Verification items for the finished model (mm, model axes). A direction names the side the tool comes from. Give positions to 0.01 mm unless a question says otherwise; leave off trailing zeros. Order: outer loops, then holes, each group sorted by start corner. A loop starts at its lowest first (then second) coordinate and runs counter-clockwise, first axis right, second up.
(1) Gauge pin test, flat end, axial feed: pin 1 (1.4 mm diameter, centred on x = -2.67, z = -1.24, fed in from -Y). Record the tip position at first contact, or that the pin passes through.
(2) Access from +Z, -Z, +X, -X, +Y, -Y to the whole of each face (thin tool, end or side, straight path). Record for faces 4 (the face through (-8, 2, -3.388)), 5 (the face through (-12.598, 2, 4)).
(3) Sectioned sample at B-B on z = 3. Record the cut outline in (x, y), plus the area to 3 significant figures.
(4) Sectioned sample at A-A on x = -9.5. Record the cut outline in (y, z), plus the area to 3 significant figures.
(5) Mould release check, pull along Z, two halves, no side actions. Record for faces 1 (the face through (-6, 5, 4)), 2 (the face through (-6, 2, -4.541)), 3 (the face through (-8.17, 2.46, 1.41)): pulls with the +Z half, pulls with the -Z half, needs draft (parallel to the pull), parting line crosses it, or undercut.
(6) Sectioned sample at C-C on y = 4.2. Record the cut outline in (x, z).
(7) Scan lines: L1, parallel to Z at x = -4, y = 3.6; L2, parallel to X at y = 2.8, z = 3.5; L3, parallel to X at y = 2.95, z = 9. Record each from-to range of solid material in increasing order.
```python
from build123d import *

# Parameters (mm, degrees)
SKETCH1_W           = 13.581948161
SKETCH1_H           = 17.761009134
SKETCH1_R           = 1.6
SKETCH1_R_2         = 1.2
SKETCH1_R_3         = 1.75
BOSS_EXTRUDE1_DEPTH = 5


with BuildPart() as part:
    # Sketch1 → Boss-Extrude1 (new body)
    with BuildSketch(Plane(origin=(0, 0, 0), x_dir=(1, 0, 0), z_dir=(0, 1, 0))):
        with Locations((-5.80679888, -4.339957405)):
            Rectangle(SKETCH1_W, SKETCH1_H)
        with Locations(Location((-2.596056365, -9.056132184, 0), (0, 0, 270))):
            Circle(SKETCH1_R, mode=Mode.SUBTRACT)
        with Locations(Location((-2.667047062, 1.237786047, 0), (0, 0, 270))):
            Circle(SKETCH1_R_2, mode=Mode.SUBTRACT)
        with Locations(Location((-3.046693025, -3.619626487, 0), (0, 0, 270))):
            Circle(SKETCH1_R_3, mode=Mode.SUBTRACT)
        with BuildLine():
            Line((-9.810909871, 3.387786047), (-6.712523194, 3.387786047))
            ThreePointArc((-6.712523194, 3.387786047), (-8.261716533, -1.412213953), (-9.810909871, 3.387786047))
        make_face(mode=Mode.SUBTRACT)
    extrude(amount=BOSS_EXTRUDE1_DEPTH)


solid = part.part
```
Ans:
1. pin 1: passes through
2. face 4: +Y, -Y
2. face 5: +Z, -Z, -X, +Y, -Y
3. outline: (-12.6, 0) - (-4.68, 0) - (-4.68, 5) - (-12.6, 5) - close; (-1.41, 0) - (0.98, 0) - (0.98, 5) - (-1.41, 5) - close
3. area: 51.5 mm2
4. outline: (0, -4.54) - (5, -4.54) - (5, -3.39) - (0, -3.39) - close; (0, 1.11) - (5, 1.11) - (5, 13.22) - (0, 13.22) - close
4. area: 66.3 mm2
5. face 1: needs draft
5. face 2: pulls with the -Z half
5. face 3: undercut
6. outline: (-12.6, -4.54) - (0.98, -4.54) - (0.98, 13.22) - (-12.6, 13.22) - close; hole (-9.81, -3.39) - (-6.71, -3.39) arc R2.65 ccw (long way) to start; hole circle Ø3.5 at (-3.05, 3.62); hole circle Ø3.2 at (-2.6, 9.06); hole circle Ø2.4 at (-2.67, -1.24)
7. L1: z = -4.54 to 2.15, 5.09 to 8.29, 9.82 to 13.22
7. L2: x = -12.6 to -4.79, -1.3 to 0.98
7. L3: x = -12.6 to -4.2, -1 to 0.98
